For this review, use the dimensioned drawing (mm, ordinates from the lowest corner) and the shaded views. A direction names the side the tool comes from. Give positions to 0.01 mm unless a question says otherwise; leave off trailing zeros. Order: outer loops, then holes, each group sorted by start corner. A loop starts at its lowest first (then second) coordinate and runs counter-clockwise, first axis right, second up.
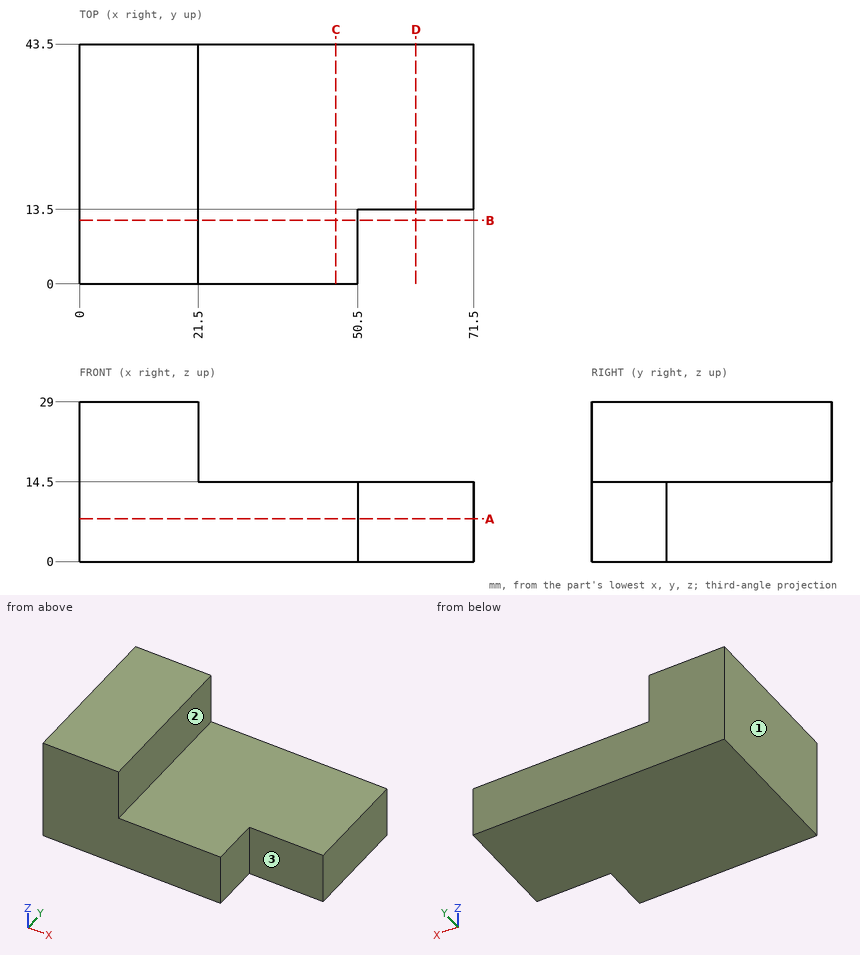
1. For line 1 along X through (y, z) = (24, 18.75); line 2 along Z through (x, y) = (27, 29); line 3 along X through (y, z) = (8.5, 10.75), list the stretches that pass through material, from the lowest coordinate up.
Recorded:
line 1: x = 0 to 21.5
line 2: z = 0 to 14.5
line 3: x = 0 to 50.5
2. Take a section at C-C (x = 46.5). State the section outline as (y, z) points.
Recorded:
outline: (0, 0) - (43.5, 0) - (43.5, 14.5) - (0, 14.5) - close
3. Take a section at A-A (z = 7.75). State the section outline as (x, y) points.
Recorded:
outline: (0, 0) - (50.5, 0) - (50.5, 13.5) - (71.5, 13.5) - (71.5, 43.5) - (0, 43.5) - close
4. Take a section at D-D (x = 61). State the section outline as (y, z) points.
Recorded:
outline: (13.5, 0) - (43.5, 0) - (43.5, 14.5) - (13.5, 14.5) - close
5. Machinability: for the marked faces 1, 2 and 3, which of the approach directions +Z, -Z, +X, -X, +Y, -Y give a long, thin tool a straight path to every point of the face, cutting with its end or side? Answer none if there is none.
Recorded:
face 1: +Z, -Z, -X, +Y, -Y
face 2: +Z, +X, +Y, -Y
face 3: +Z, -Z, +X, -Y
6. Take a section at B-B (y = 11.5). State the section outline as (x, z) points.
Recorded:
outline: (0, 0) - (50.5, 0) - (50.5, 14.5) - (21.5, 14.5) - (21.5, 29) - (0, 29) - close
7. For pin 1 (5 mm diameter, centred on x = 59.5, y = 20, fed in from +Z); pin 2 (11.5 mm diameter, centred on x = 63.5, z = 4, fed in from -Y); pin 3 (15 mm diameter, centred on y = 4.5, z = 4.5, fed in from +X), all flat-tipped, find the tip position at first contact; note any pin that passes through.
Recorded:
pin 1: stops at z = 14.5
pin 2: stops at y = 13.5
pin 3: stops at x = 50.5
